The listing builds one solid part. Answer for the finished solid, in the listing's coordinates (mm). Face numbers are marked on the shaded views. A direction names the side the tool comes from. Give positions to 0.01 mm unless a question says otherwise; leave off trailing zeros. Order: outer loops, then holes, each group sorted by start corner. A loop starts at its lowest first (then second) coordinate and runs counter-clockwise, first axis right, second up. Notation, with made-up numbers: (85.25, 20) - (99.25, 20) arc R19 ccw to (99.25, 56) - close; hole circle Ø10 at (22, 3). An arc over 180 degrees is marked (long way). Answer as a JSON object with one key per item and string values. Group by question number.
Q1. Given pin 1 (3 mm diameter, centred on x = 11.46, z = -10.05, fed in from +Y); pin 2 (10 mm diameter, centred on x = 49.5, y = 44.5, fed in from -Z); pin 3 (10.5 mm diameter, centred on x = 20, y = 44, fed in from -Z); pin 4 (4.5 mm diameter, centred on x = 58.54, z = -10.05, fed in from +Y), each flat-ended and moving along its own axis, determine where each tip first touches the part or whether it passes through.
Q2. The mould has two halves that part along X. Classify the marked faces 1, 2 and 3: released by +X, released by -X, zero draft, split by the parting line, or undercut.
Q3. A cutting plane is placed at A-A, the plane x = 35. Give the vertices of the cut face in (y, z), and give its area (4 significant figures).
Q4. For the marked faces 4 and 5, determine the directions among +Z, -Z, +X, -X, +Y, -Y from which every point of the face is accessible in a straight line to the end or side of a thin tool.
Q5. A cutting plane is placed at D-D, the plane x = 20. Give the vertices of the cut face in (y, z).
Q6. A cutting plane is placed at B-B, the plane z = -33.2. Give the vertices of the cut face in (x, y), and give its area (3 significant figures).
Q7. Consider line 1 (Y direction, x = 20, z = -1.4); line 2 (X direction, y = 64, z = -1.25); line 3 (X direction, y = 63.5, z = -17.5). Determine where each line is inside the solid, lowest interval first.
Q8. A cutting plane is placed at C-C, the plane y = 24. Give the vertices of the cut face in (x, z).
from build123d import *

# Parameters (mm, degrees)
DODANIE_WYCI_GNI_CIE1_DEPTH              = 70
DODANIE_WYCI_GNI_CIE2_DEPTH              = 6.8
OTW_R_GWINTOWANY_M41_D                   = 3.3
SZKIC3_R                                 = 19.05
WYTNIJ_WYCI_GNI_CIE1_DEPTH               = 9.8
POG_BIENIE_STO_KOWE_POD_M6_RUB_Z_2_COUNT = 2
POG_BIENIE_STO_KOWE_POD_M6_RUB_Z_2_PITCH = 30
POG_BIENIE_STO_KOWE_POD_M6_RUB_Z_3_COUNT = 2
POG_BIENIE_STO_KOWE_POD_M6_RUB_Z_3_PITCH = 20
POG_BIENIE_STO_KOWE_POD_M6_RUB_Z_4_COUNT = 2
POG_BIENIE_STO_KOWE_POD_M6_RUB_Z_4_PITCH = 36.055512755
POG_BIENIE_STO_KOWE_POD_M6_RUB_Z_5_COUNT = 2
POG_BIENIE_STO_KOWE_POD_M6_RUB_Z_5_PITCH = 40
POG_BIENIE_STO_KOWE_POD_M6_RUB_Z_6_COUNT = 2
POG_BIENIE_STO_KOWE_POD_M6_RUB_Z_6_PITCH = 50


with BuildPart() as part:
    # Szkic1 → Dodanie-wyciągnięcie1 (new body)
    with BuildSketch(Plane(origin=(0, 0, 0), x_dir=(0, 0, -1), z_dir=(1, 0, 0))):
        Polygon((0, 0), (61.4, 0), (61.4, 5), (5, 5), (5, 81), (0, 81), align=None)
    extrude(amount=DODANIE_WYCI_GNI_CIE1_DEPTH)

    # Szkic2 → Dodanie-wyciągnięcie2 (add)
    with BuildSketch(Plane(origin=(70, 0, 0), x_dir=(0, 0, -1), z_dir=(1, 0, 0))):
        Polygon((5, 81), (61.4, 5), (5, 5), align=None)
    dodanie_wyci_gni_cie2 = extrude(amount=-DODANIE_WYCI_GNI_CIE2_DEPTH)

    # Lustro1: Dodanie-wyciągnięcie2 across plane
    add(dodanie_wyci_gni_cie2.mirror(Plane(origin=(35, 0, 0), x_dir=(0, 0, 1), z_dir=(1, 0, 0))))

    # Otwór gwintowany M41 (through all)
    with Locations(Plane(origin=(11.455, 5, -57.137511403), x_dir=(0, 0, 1), z_dir=(0, 1, 0))):
        with Locations((0, 0), (0, 47.09), (47.09, 0), (47.09, 47.09)):
            Hole(OTW_R_GWINTOWANY_M41_D / 2)

    # Szkic3 → Wytnij-wyciągnięcie1 (cut)
    with BuildSketch(Plane(origin=(0, 5, 0), x_dir=(1, 0, 0), z_dir=(0, 1, 0))):
        with Locations(Location((35, 33.2, 0), (0, 0, 270))):
            Circle(SZKIC3_R)
    extrude(amount=-WYTNIJ_WYCI_GNI_CIE1_DEPTH, mode=Mode.SUBTRACT)

    # Szkic7 → Pogłębienie stożkowe pod M6 Śrubę z łbem soczewkowym1 (revolve, cut)
    with BuildSketch(Plane(origin=(50, 64, -5), x_dir=(0, 1, 0), z_dir=(1, 0, 0))):
        Polygon((0, 0), (0, 5), (3.3, 5), (3.3, 3), (6.3, 0), align=None)
    pog_bienie_sto_kowe_pod_m6_rub_z_bem = revolve(axis=Axis((50, 64, -11.35), (0, 0, 1)), mode=Mode.SUBTRACT)

    # Pog_bienie sto_kowe pod M6 _rub_ z _ 2: Pogłębienie stożkowe pod M6 Śrubę z łbem soczewkowym1 ×2
    with Locations(*[(-i * POG_BIENIE_STO_KOWE_POD_M6_RUB_Z_2_PITCH, 0, 0) for i in range(1, POG_BIENIE_STO_KOWE_POD_M6_RUB_Z_2_COUNT)]):
        add(pog_bienie_sto_kowe_pod_m6_rub_z_bem, mode=Mode.SUBTRACT)

    # Pog_bienie sto_kowe pod M6 _rub_ z _ 3: Pogłębienie stożkowe pod M6 Śrubę z łbem soczewkowym1 ×2
    with Locations(*[(0, -i * POG_BIENIE_STO_KOWE_POD_M6_RUB_Z_3_PITCH, 0) for i in range(1, POG_BIENIE_STO_KOWE_POD_M6_RUB_Z_3_COUNT)]):
        add(pog_bienie_sto_kowe_pod_m6_rub_z_bem, mode=Mode.SUBTRACT)

    # Pog_bienie sto_kowe pod M6 _rub_ z _ 4: Pogłębienie stożkowe pod M6 Śrubę z łbem soczewkowym1 ×2
    with Locations(*[Vector(-0.8320502943378438, -0.5547001962252289, 0) * (i * POG_BIENIE_STO_KOWE_POD_M6_RUB_Z_4_PITCH) for i in range(1, POG_BIENIE_STO_KOWE_POD_M6_RUB_Z_4_COUNT)]):
        add(pog_bienie_sto_kowe_pod_m6_rub_z_bem, mode=Mode.SUBTRACT)

    # Pog_bienie sto_kowe pod M6 _rub_ z _ 5: Pogłębienie stożkowe pod M6 Śrubę z łbem soczewkowym1 ×2
    with Locations(*[(0, -i * POG_BIENIE_STO_KOWE_POD_M6_RUB_Z_5_PITCH, 0) for i in range(1, POG_BIENIE_STO_KOWE_POD_M6_RUB_Z_5_COUNT)]):
        add(pog_bienie_sto_kowe_pod_m6_rub_z_bem, mode=Mode.SUBTRACT)

    # Pog_bienie sto_kowe pod M6 _rub_ z _ 6: Pogłębienie stożkowe pod M6 Śrubę z łbem soczewkowym1 ×2
    with Locations(*[Vector(-0.6000000000000001, -0.7999999999999999, 0) * (i * POG_BIENIE_STO_KOWE_POD_M6_RUB_Z_6_PITCH) for i in range(1, POG_BIENIE_STO_KOWE_POD_M6_RUB_Z_6_COUNT)]):
        add(pog_bienie_sto_kowe_pod_m6_rub_z_bem, mode=Mode.SUBTRACT)


solid = part.part
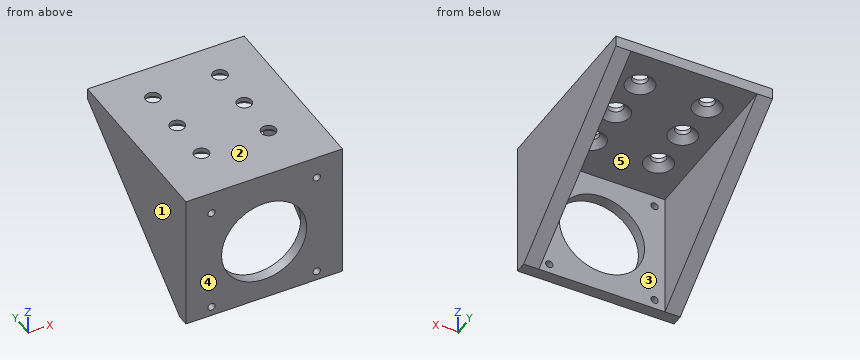
Reply:
{
 "1": {"pin 1": "passes through", "pin 2": "stops at z = -4.41", "pin 3": "stops at z = -3.95", "pin 4": "stops at y = 5"},
 "2": {"face 1": "released by -X", "face 2": "zero draft", "face 3": "undercut"},
 "3": {"outline": "(0, -61.4) - (5, -61.4) - (5, -52.25) - (0, -52.25) - close; (0, -14.15) - (5, -14.15) - (5, -5) - (81, -5) - (81, 0) - (0, 0) - close", "area": "496.5 mm^2"},
 "4": {"face 4": "+Z, -Z, +X, -X, -Y", "face 5": "-Z, +Y"},
 "5": {"outline": "(0, -61.4) - (5, -61.4) - (5, -44.94) - (0, -44.94) - close; (0, -21.46) - (5, -21.46) - (5, -5) - (17.7, -5) - (20.7, -2) - (20.7, 0) - (0, 0) - close; (27.3, -2) - (30.3, -5) - (37.7, -5) - (40.7, -2) - (40.7, 0) - (27.3, 0) - close; (47.3, -2) - (50.3, -5) - (57.7, -5) - (60.7, -2) - (60.7, 0) - (47.3, 0) - close; (67.3, -2) - (70.3, -5) - (81, -5) - (81, 0) - (67.3, 0) - close"},
 "6": {"outline": "(0, 0) - (15.95, 0) - (15.95, 5) - (6.8, 5) - (6.8, 43) - (0, 43) - close; (54.05, 0) - (70, 0) - (70, 43) - (63.2, 43) - (63.2, 5) - (54.05, 5) - close", "area": "676 mm^2"},
 "7": {"line 1": "y = 0 to 20.7, 27.3 to 40.7, 47.3 to 60.7, 67.3 to 81", "line 2": "x = 0 to 16.7, 23.3 to 46.7, 53.3 to 70", "line 3": "x = 0 to 6.8, 63.2 to 70"},
 "8": {"outline": "(0, -47.3) - (6.8, -47.3) - (6.8, -5) - (13.7, -5) - (16.7, -2) - (16.7, 0) - (0, 0) - close; (23.3, -2) - (26.3, -5) - (43.7, -5) - (46.7, -2) - (46.7, 0) - (23.3, 0) - close; (53.3, -2) - (56.3, -5) - (63.2, -5) - (63.2, -47.3) - (70, -47.3) - (70, 0) - (53.3, 0) - close"}
}
